Geometry check sheet. Reference: the model listing, model coordinates, mm. A direction names the side the tool comes from. Round coordinates to 2 decimals unless told otherwise and drop trailing zeros. Write each loop counter-clockwise with the first axis right and the second up, starting at its lowest first coordinate (ties: lowest second). Pieces come first, ordered by that corner, then holes.
Item 1: Cross-section at D-D (x = 9). Enter the section's corners in (y, z) (3 decimals), then the cut area to 3 significant figures.
Item 2: Cross-section at A-A (y = 0). Enter the section's corners in (x, z), then the cut area to 3 significant figures.
Item 3: Draft check along X on faces 3 (the face through (1.374, 12.108, 2.504)), 4 (the face through (-6.883, -30.995, 2.504)), 5 (the face through (-14.6, -6.6, 5.08)). Enter one of: pulls with the +X half, pulls with the -X half, needs draft (parallel to the pull), parting line crosses it, or undercut.
Item 4: Depth check by flat-ended pin: P1, Ø8, axis at x = -6.5, z = 18, coming from the -Y side; P2, Ø2, axis at y = -6.5, z = 22.5, coming from the +X side; P3, Ø1.5, axis at x = 9.5, z = 16.5, coming from the +Y side. Enter the tip coordinate at first touch or a pass-through.
Item 5: Access from +Z, -Z, +X, -X, +Y, -Y to the whole of each face (thin tool, end or side, straight path). Record for faces 1 (the face through (8.43, -0.95, 24.88)), 2 (the face through (-10.902, -3.433, 19.355)).
Item 6: Scan lines: probe 1 along X at (y, z) = (-10.5, 4); probe 2 along Z at (x, y) = (26, -7); probe 3 along X at (y, z) = (10, 2). Record each from-to range of solid material in increasing order.
Item 7: Cross-section at C-C (y = -21.5). Enter the section's corners in (x, z), then the cut area to 3 significant figures.
Item 8: Cross-section at B-B (x = 0). Enter the section's corners in (y, z), then the cut area to 3 significant figures.
from build123d import *

# Parameters (mm, degrees)
SKETCH1_R               = 31.75
BOSS_EXTRUDE1_DEPTH     = 5.08
SKETCH2_R               = 6.35
CUT_EXTRUDE1_DEPTH      = 5.08
SKETCH3_R               = 11.43
BOSS_EXTRUDE2_DEPTH     = 28.956
CUT_EXTRUDE2_START      = -29.21
SKETCH5_R               = 6.35
CUT_EXTRUDE2_DEPTH      = 29.21
SKETCH6_R               = 6.337124867
CUT_EXTRUDE3_DEPTH      = 5.08
CUT_EXTRUDE4_DEPTH      = 17.526
CUT_EXTRUDE4_DEPTH_BACK = 11.938
SKETCH7_R               = 3.175


with BuildPart() as part:
    # Sketch1 → Boss-Extrude1 (new body)
    with BuildSketch(Plane.XY):
        Circle(SKETCH1_R)
    extrude(amount=BOSS_EXTRUDE1_DEPTH)

    # Sketch2 → Cut-Extrude1 (cut)
    with BuildSketch(Plane(origin=(0, 0, 0), x_dir=(-1, 0, 0), z_dir=(0, 0, -1))):
        Circle(SKETCH2_R)
    extrude(amount=-CUT_EXTRUDE1_DEPTH, mode=Mode.SUBTRACT)

    # Sketch3 → Boss-Extrude2 (add)
    with BuildSketch(Plane.XY.offset(5.08)):
        with Locations(Location((0, 0, 0), (0, 0, 180))):
            Circle(SKETCH3_R)
    extrude(amount=BOSS_EXTRUDE2_DEPTH)

    # Sketch5 → Cut-Extrude2 (cut)
    with BuildSketch(Plane.XY.offset(34.036).offset(CUT_EXTRUDE2_START)):
        with Locations(Location((0, 0, 0), (0, 0, 180))):
            Circle(SKETCH5_R)
    extrude(amount=CUT_EXTRUDE2_DEPTH, mode=Mode.SUBTRACT)

    # Sketch6 → Cut-Extrude3 (cut)
    with BuildSketch(Plane(origin=(0, 0, 0), x_dir=(-1, 0, 0), z_dir=(0, 0, -1))):
        with Locations((0, 18.294370769)):
            Circle(SKETCH6_R)
        with Locations((12.936073628, 12.936073628)):
            Circle(SKETCH6_R)
        with Locations((18.294370769, 0)):
            Circle(SKETCH6_R)
        with Locations((12.936073628, -12.936073628)):
            Circle(SKETCH6_R)
        with Locations((0, -18.294370769)):
            Circle(SKETCH6_R)
        with Locations((-12.936073628, -12.936073628)):
            Circle(SKETCH6_R)
        with Locations((-18.294370769, 0)):
            Circle(SKETCH6_R)
        with Locations((-12.936073628, 12.936073628)):
            Circle(SKETCH6_R)
    extrude(amount=-CUT_EXTRUDE3_DEPTH, mode=Mode.SUBTRACT)

    # Sketch7 → Cut-Extrude4 (cut, two sides: drawn at the far end of the back side and taken through both)
    with BuildSketch(Plane(origin=(0, 0, 0), x_dir=(0, 0, -1), z_dir=(1, 0, 0)).offset(-CUT_EXTRUDE4_DEPTH_BACK)):
        with Locations(Location((-21.851313678, 0, 0), (0, 0, 180))):
            Circle(SKETCH7_R)
    extrude(amount=CUT_EXTRUDE4_DEPTH + CUT_EXTRUDE4_DEPTH_BACK, mode=Mode.SUBTRACT)


solid = part.part
Resolved:
1. outline: (-30.448, 0) - (-17.903, 0) - (-17.903, 5.08) - (-30.448, 5.08) - close; (-7.97, 0) - (7.97, 0) - (7.97, 5.08) - (7.046, 5.08) - (7.046, 34.036) - (-7.046, 34.036) - (-7.046, 5.08) - (-7.97, 5.08) - close; (17.903, 0) - (30.448, 0) - (30.448, 5.08) - (17.903, 5.08) - close; hole circle Ø6.35 at (0, 21.851)
1. area: 585 mm2
2. outline: (-31.75, 0) - (-24.63, 0) - (-24.63, 5.08) - (-31.75, 5.08) - close; (-11.96, 0) - (-6.35, 0) - (-6.35, 18.68) - (-11.43, 18.68) - (-11.43, 5.08) - (-11.96, 5.08) - close; (-11.43, 25.03) - (-6.35, 25.03) - (-6.35, 34.04) - (-11.43, 34.04) - close; (6.35, 0) - (11.96, 0) - (11.96, 5.08) - (11.43, 5.08) - (11.43, 18.68) - (6.35, 18.68) - close; (6.35, 25.03) - (11.43, 25.03) - (11.43, 34.04) - (6.35, 34.04) - close; (24.63, 0) - (31.75, 0) - (31.75, 5.08) - (24.63, 5.08) - close
2. area: 359 mm2
3. face 3: undercut
3. face 4: parting line crosses it
3. face 5: needs draft
4. P1: stops at y = -11.15
4. P2: stops at x = 10.02
4. P3: stops at y = 7.35
5. face 1: +X, -X
5. face 2: +Z
6. probe 1: x = -29.96 to -18.79, -7.09 to 7.09, 18.79 to 29.96
6. probe 2: z = 0 to 5.08
6. probe 3: x = -30.13 to -18.55, -7.32 to 7.32, 18.55 to 30.13
7. outline: (-23.36, 0) - (-5.47, 0) - (-5.47, 5.08) - (-23.36, 5.08) - close; (5.47, 0) - (23.36, 0) - (23.36, 5.08) - (5.47, 5.08) - close
7. area: 182 mm2
8. outline: (-31.75, 0) - (-24.63, 0) - (-24.63, 5.08) - (-31.75, 5.08) - close; (-11.96, 0) - (-6.35, 0) - (-6.35, 34.04) - (-11.43, 34.04) - (-11.43, 5.08) - (-11.96, 5.08) - close; (6.35, 0) - (11.96, 0) - (11.96, 5.08) - (11.43, 5.08) - (11.43, 34.04) - (6.35, 34.04) - close; (24.63, 0) - (31.75, 0) - (31.75, 5.08) - (24.63, 5.08) - close
8. area: 423 mm2
